Geometry: final body of the model. Coordinates: model frame, mm. Face numbers are marked on the shaded views. Give positions to 0.01 mm unless a question says otherwise; leave off trailing zeros. Write each loop counter-clockwise with the first axis right and the second up, starting at its lowest first coordinate (ties: lowest second). Pieces come first, ordered by that corner, then holes. Notation, with made-up numbers: M 67.5,85.25 L 76.5,85.25 A23 ccw 76.5,107.25 Z; hole C 54.5,59.25 d1. An arc over 180 degrees is marked long. Use one line per item in the form item = value. Start each with the question number.
Item 1: Contact query for flat-ended pins moving along their axis: P1, Ø11.5, axis at x = 0, y = 0, coming from the -Z side; P2, Ø11, axis at x = -127, y = 0, coming from the +Z side; P3, Ø10, axis at y = -72.5, z = -15, coming from the +X side; P4, Ø2, axis at x = -27, z = -9.5, coming from the +Y side. Output: stop coordinate, or through.
Item 2: Section query A-A on y = 0. Return loops of the section in (x, z) (3 decimals).
Item 3: Section query B-B on x = 0. Return loops of the section in (y, z), then the cut area to 3 significant figures.
Item 4: Section query C-C on z = -34. Return loops of the section in (x, y).
Item 5: Pull-direction query (X, two-part tool) for the marked faces 1, 2 and 3; classes: released by +X, released by -X, zero draft, split by the parting line, or undercut.
Item 6: Material intervals for line 1 along X through (y, z) = (0, -20); line 2 along Z through (x, y) = (-39, 19.5), sorted ascending. Write a range as from..to.
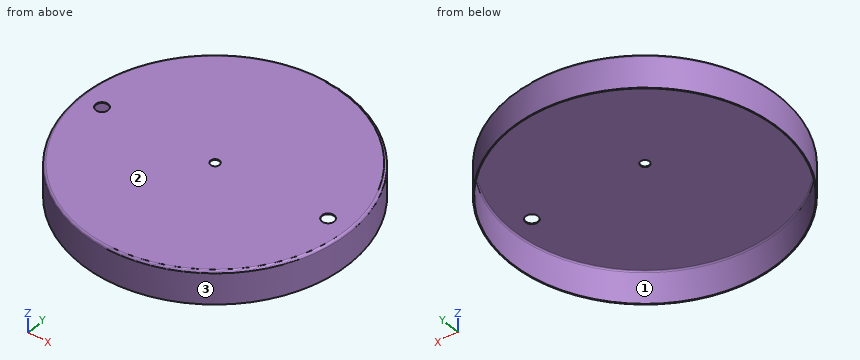
from build123d import *

# Parameters (mm, degrees)
F3_R     = 6.985
F3_R_2   = 5.08
F4_DEPTH = 1.016


with BuildPart() as f2:
    # F1 (on Front) → F2 (revolve)
    with BuildSketch(Plane.XZ):
        with BuildLine():
            Line((149.86, 0), (0, 0))
            Line((0, 0), (0, -1.016))
            Line((0, -1.016), (149.86, -1.016))
            ThreePointArc((149.86, -1.016), (150.937631, -1.462369), (151.384, -2.54))
            Line((151.384, -2.54), (151.384, -38.1))
            Line((151.384, -38.1), (152.4, -38.1))
            Line((152.4, -38.1), (152.4, -2.54))
            ThreePointArc((152.4, -2.54), (151.656051, -0.743949), (149.86, 0))
        make_face()
    revolve(axis=Axis((0, 0, -9.205109), (0, 0, -1)))

    # F3 (on face) → F4 (cut, through all)
    with BuildSketch(Plane.XY):
        with Locations((127, 0)):
            Circle(F3_R)
        with Locations((-127, 0)):
            Circle(F3_R)
        Circle(F3_R_2)
    extrude(amount=-F4_DEPTH, mode=Mode.SUBTRACT)


solid = f2.part
Answer sheet:
q1.P1 = -1.02
q1.P2 = through
q1.P3 = 136.64
q1.P4 = 150.17
q2.outline = M -152.4,-38.1 L -151.384,-38.1 L -151.384,-2.54 A1.524 cw -149.86,-1.016 L -133.985,-1.016 L -133.985,0 L -149.86,0 A2.54 ccw -152.4,-2.54 Z; M -120.015,-1.016 L -5.08,-1.016 L -5.08,0 L -120.015,0 Z; M 5.08,-1.016 L 120.015,-1.016 L 120.015,0 L 5.08,0 Z; M 133.985,-1.016 L 149.86,-1.016 A1.524 cw 151.384,-2.54 L 151.384,-38.1 L 152.4,-38.1 L 152.4,-2.54 A2.54 ccw 149.86,0 L 133.985,0 Z
q3.outline = M -152.4,-38.1 L -151.38,-38.1 L -151.38,-2.54 A1.52 cw -149.86,-1.02 L -5.08,-1.02 L -5.08,0 L -149.86,0 A2.54 ccw -152.4,-2.54 Z; M 5.08,-1.02 L 149.86,-1.02 A1.52 cw 151.38,-2.54 L 151.38,-38.1 L 152.4,-38.1 L 152.4,-2.54 A2.54 ccw 149.86,0 L 5.08,0 Z
q3.area = 373 mm2
q4.outline = C 0,0 d304.8; hole C 0,0 d302.77
q5.face_1 = undercut
q5.face_2 = zero draft
q5.face_3 = split by the parting line
q6.line_1 = -152.4..-151.38, 151.38..152.4
q6.line_2 = -1.02..0
